The listing builds one solid part. Answer for the finished solid, in the listing's coordinates (mm). Give positions to 0.01 mm unless a question says otherwise; leave off trailing zeros. Loops run counter-clockwise (first coordinate to the right, second up) from the corner with the lowest first, then second, coordinate; pieces in that order, holes last. Notation, with made-up numbers: (-14.75, 81) - (27.25, 81) arc R24 cw to (27.25, 93) - close; hole circle Ø5 at (32, 48). An arc over 180 degrees is marked (long way). Write each question's results on one line, items separated by ' | '.
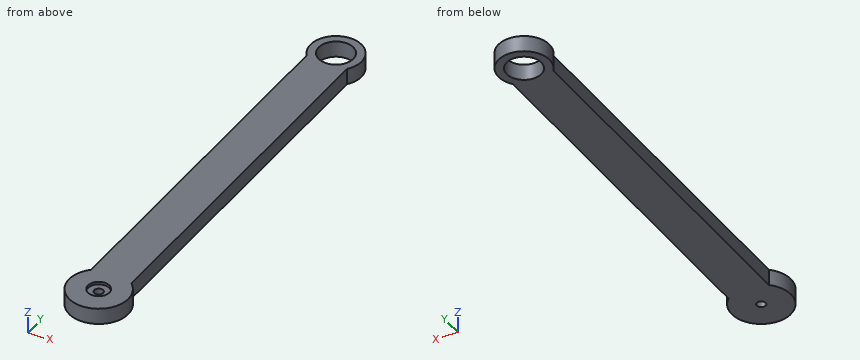
from build123d import *

# Parameters (mm, degrees)
ESQUISSE1_W             = 15
ESQUISSE1_H             = 165
BOSS_EXTRU_1_DEPTH      = 6
ESQUISSE2_R             = 11
ESQUISSE2_R_2           = 9.5
BOSS_EXTRU_2_DEPTH      = 6
ESQUISSE3_R             = 1.65
ESQUISSE3_R_2           = 6.45
ENL_V_MAT_EXTRU_1_DEPTH = 10
ESQUISSE4_R             = 4
ENL_V_MAT_EXTRU_2_DEPTH = 1


with BuildPart() as part:
    # Esquisse1 → Boss.-Extru.1 (new body)
    with BuildSketch(Plane.XY):
        with Locations((7.5, 82.5)):
            Rectangle(ESQUISSE1_W, ESQUISSE1_H)
    extrude(amount=BOSS_EXTRU_1_DEPTH)

    # Esquisse2 → Boss.-Extru.2 (add)
    with BuildSketch(Plane.XY.offset(6)):
        with Locations((7.5, 7.5)):
            Circle(ESQUISSE2_R)
        with Locations((7.5, 159.25)):
            Circle(ESQUISSE2_R_2)
    extrude(amount=-BOSS_EXTRU_2_DEPTH)

    # Esquisse3 → Enlèv. mat.-Extru.1 (cut)
    with BuildSketch(Plane(origin=(0, 0, 0), x_dir=(-1, 0, 0), z_dir=(0, 0, -1))):
        with Locations((-7.5, 7.5)):
            Circle(ESQUISSE3_R)
        with Locations((-7.5, 159.25)):
            Circle(ESQUISSE3_R_2)
    extrude(amount=-ENL_V_MAT_EXTRU_1_DEPTH, mode=Mode.SUBTRACT)

    # Esquisse4 → Enlèv. mat.-Extru.2 (cut)
    with BuildSketch(Plane.XY.offset(6)):
        with Locations((7.5, 7.5)):
            Circle(ESQUISSE4_R)
    extrude(amount=-ENL_V_MAT_EXTRU_2_DEPTH, mode=Mode.SUBTRACT)


solid = part.part
Item 1: A cutting plane is placed at B-B, the plane y = 7.5. Determine the outline of the cut face in (x, z), plus the area to 4 significant figures.
Values found:
outline: (-3.5, 0) - (5.85, 0) - (5.85, 5) - (3.5, 5) - (3.5, 6) - (-3.5, 6) - close; (9.15, 0) - (18.5, 0) - (18.5, 6) - (11.5, 6) - (11.5, 5) - (9.15, 5) - close | area: 107.5 mm²
Item 2: A cutting plane is placed at C-C, the plane z = 4.05. Determine the outline of the cut face in (x, y), plus the area to 3 significant figures.
Values found:
outline: (0, 15.55) arc R11 ccw (long way) to (15, 15.55) - (15, 153.42) arc R9.5 ccw (long way) to (0, 153.42) - close; hole circle Ø12.9 at (7.5, 159.25); hole circle Ø3.3 at (7.5, 7.5) | area: 2,520 mm²
Item 3: A cutting plane is placed at A-A, the plane x = 7.5. Determine the outline of the cut face in (y, z), plus the area to 3 significant figures.
Values found:
outline: (-3.5, 0) - (5.85, 0) - (5.85, 5) - (3.5, 5) - (3.5, 6) - (-3.5, 6) - close; (9.15, 0) - (152.8, 0) - (152.8, 6) - (11.5, 6) - (11.5, 5) - (9.15, 5) - close; (165.7, 0) - (168.75, 0) - (168.75, 6) - (165.7, 6) - close | area: 932 mm²
Item 4: Flat-ended cylindrical pins translate along their axes: P1, Ø1.5, axis at x = 14.5, z = 4.5, coming from the +Y side; P2, Ø1.5, axis at y = 128.5, z = 1.5, coming from the -X side; P3, Ø9, axis at x = 6, y = 9, coming from the +Z side; P4, Ø3, axis at y = 55, z = 3, coming from the +X side. Find the tip coordinate at first contact, or state that the pin passes through.
Values found:
P1: stops at y = 166.4 | P2: stops at x = 0 | P3: stops at z = 6 | P4: stops at x = 15
Item 5: A cutting plane is placed at D-D, the plane y = 159.25. Determine the outline of the cut face in (x, z).
Values found:
outline: (-2, 0) - (1.05, 0) - (1.05, 6) - (-2, 6) - close; (13.95, 0) - (17, 0) - (17, 6) - (13.95, 6) - close
Item 6: Find the intervals of material crossed by line 1 along Y through (x, z) = (7.5, 1.55); line 2 along Y through (x, z) = (7.5, 5.55); line 3 along X through (y, z) = (152.5, 1.35), in increasing order. Write a range as [from, to].
Values found:
line 1: y = [-3.5, 5.85], [9.15, 152.8], [165.7, 168.75] | line 2: y = [-3.5, 3.5], [11.5, 152.8], [165.7, 168.75] | line 3: x = [0, 15]
